Work out the finished part from the listing and answer in its coordinate system (mm). Face numbers are marked on the shaded views. A direction names the side the tool comes from. Round coordinates to 2 decimals unless told otherwise and drop trailing zeros. Order: outer loops, then holes, each group sorted by start corner. A loop starts at its lowest first (then second) coordinate and runs counter-clockwise, first axis right, second up. Notation, with made-up numbers: (49, -38) -> (64, -38) arc R25 ccw to (64, -2) -> close; hole circle Ø3 at (-19, -10.5). An arc over 180 degrees is marked (long way). Use a Markdown table: item, result. Add a question column.
Item 1: Find the intervals of material crossed by L1, parallel to Y at x = -0.25, z = -77.5; L2, parallel to Y at x = 1.5, z = -44; L3, parallel to X at y = 5, z = -51, in increasing order. Write a range as [from, to].
Item 2: A cutting plane is placed at A-A, the plane z = -77. Determine the outline of the cut face in (x, y).
Item 3: A tool of negligible diameter and unlimited length cuts with its end or side. For the marked faces 1, 2 and 3, from which of +Z, -Z, +X, -X, +Y, -Y can it reach the whole face along a straight path? Write none if from no direction.
Item 4: Flat-ended cylindrical pins translate along their axes: P1, Ø1.5, axis at y = 3.5, z = -89, coming from the -X side; P2, Ø4, axis at y = -4, z = -19, coming from the +X side; P3, Ø4, axis at x = 0.5, z = -63, coming from the -Y side. Find the tip coordinate at first contact, or state that the pin passes through.
Item 5: A cutting plane is placed at B-B, the plane z = -55.5. Determine the outline of the cut face in (x, y).
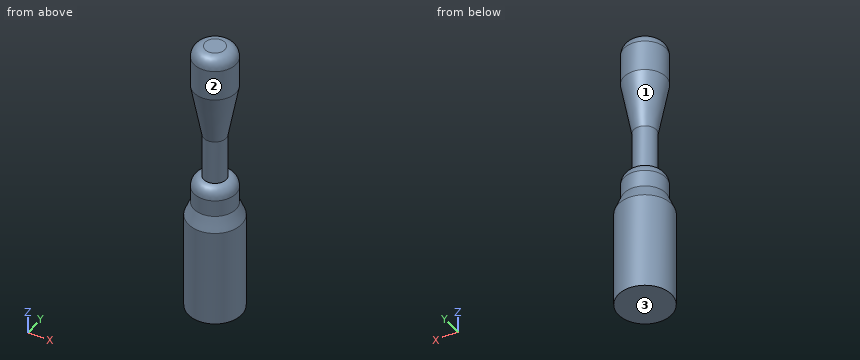
from build123d import *


with BuildPart() as f1:
    # F0 (on Front) → F1 (revolve)
    with BuildSketch(Plane.XZ):
        with BuildLine():
            Line((3.5, 0), (0, 0))
            Line((0, 0), (0, -100))
            Line((0, -100), (9.5, -100))
            Line((9.5, -100), (9.5, -65))
            Line((9.5, -65), (7.5, -60))
            Line((7.5, -60), (7.5, -54))
            ThreePointArc((7.5, -54), (6.328427, -51.171573), (3.5, -50))
            Line((3.5, -50), (4, -50))
            Line((4, -50), (4, -34))
            Line((4, -34), (7.5, -15))
            Line((7.5, -15), (7.5, -4))
            ThreePointArc((7.5, -4), (6.328427, -1.171573), (3.5, 0))
        make_face()
    revolve(axis=Axis((0, 0, -50), (0, 0, 1)))


solid = f1.part
Reported:
| question | item | result |
|---|---|---|
| 1 | L1 | [-9.5, 9.5] |
| 1 | L2 | [-3.71, 3.71] |
| 1 | L3 | [-3.57, 3.57] |
| 2 | outline | circle Ø19 at (0, 0) |
| 3 | face 1 | none |
| 3 | face 2 | +Z |
| 3 | face 3 | -Z, +X, -X, +Y, -Y |
| 4 | P1 | x = -9.09 |
| 4 | P2 | x = 6.57 |
| 4 | P3 | y = -9.49 |
| 5 | outline | circle Ø15 at (0, 0) |
